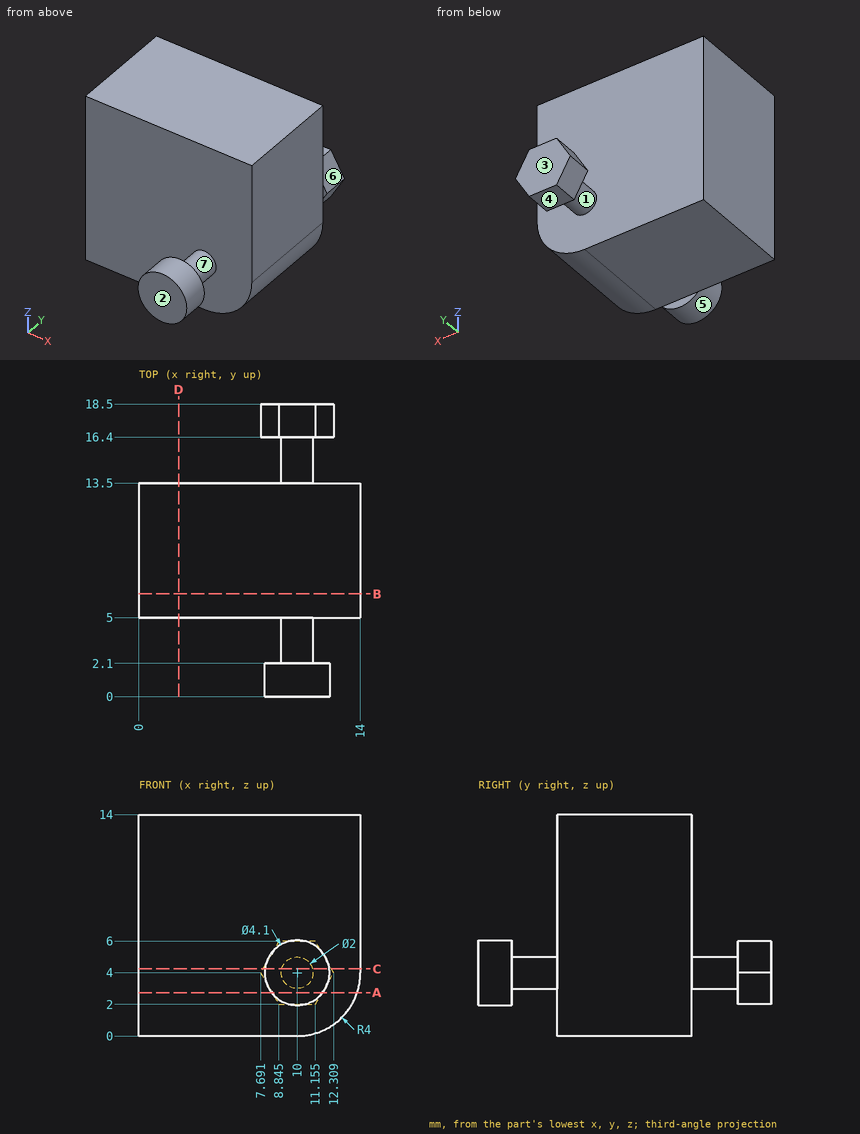
For this review, use the dimensioned drawing (mm, ordinates from the lowest corner) and the shaded views. A direction names the side the tool comes from. Round coordinates to 2 decimals unless told otherwise and drop trailing zeros. Write each loop counter-clockwise with the first axis right and the second up, starting at its lowest first coordinate (ties: lowest second). Pieces come first, ordered by that corner, then holes. Notation, with made-up numbers: (57.25, -21.5) -> (110.25, -21.5) arc R14 ccw to (110.25, -14.5) -> close; hole circle Ø11 at (-39, -23). An arc over 180 degrees is marked (long way). Answer in a Markdown table with one row per item.
Q1. Take a section at D-D, the plane x = 2.5. State the section outline as (y, z) points.
The answers:
| item | result |
|---|---|
| outline | (5, 0) -> (13.5, 0) -> (13.5, 14) -> (5, 14) -> close |
Q2. Take a section at B-B, the plane y = 6.5. State the section outline as (x, z) points, then the cut area to 3 significant figures.
The answers:
| item | result |
|---|---|
| outline | (0, 0) -> (10, 0) arc R4 ccw to (14, 4) -> (14, 14) -> (0, 14) -> close |
| area | 193 mm² |
Q3. Take a section at A-A, the plane z = 2.75. State the section outline as (x, y) points (1 decimal), then the cut area to 3 significant figures.
The answers:
| item | result |
|---|---|
| outline | (0, 5) -> (13.8, 5) -> (13.8, 13.5) -> (0, 13.5) -> close; (8.4, 0) -> (11.6, 0) -> (11.6, 2.1) -> (8.4, 2.1) -> close; (8.4, 16.4) -> (11.6, 16.4) -> (11.6, 18.5) -> (8.4, 18.5) -> close |
| area | 131 mm² |
Q4. Draft analysis for pull direction Y (two halves, no side actions). For the marked faces 1, 2 and 3, state which applies: +Y half, -Y half, draft (parallel to the pull), parting line (faces both ways), or undercut.
The answers:
| item | result |
|---|---|
| face 1 | undercut |
| face 2 | -Y half |
| face 3 | +Y half |
Q5. Clearance check with flat-ended pins moving along their axes: pin 1 Ø1.5 at (y, z) = (11.5, 2.5) entering from -X; pin 2 Ø3 at (x, y) = (9, 2) entering from -Z; pin 3 Ø1.1 at (x, y) = (10.5, 17) entering from +Z; pin 4 Ø4 at (x, z) = (4.5, 7.5) entering from +Y. State where each tip first meets the part, or that it passes through.
The answers:
| item | result |
|---|---|
| pin 1 | x = 0 |
| pin 2 | z = 1.95 |
| pin 3 | z = 6 |
| pin 4 | y = 13.5 |
Q6. To check wall thickness, follow L1, parallel to Y at x = 12.25, z = 4.5; L2, parallel to X at y = 13.25, z = 3.5; L3, parallel to Z at x = 10.25, y = 11.75. State the ranges of each line that lie inside material, in increasing order. Write a range as [from, to].
The answers:
| item | result |
|---|---|
| L1 | [5, 13.5] |
| L2 | [0, 13.97] |
| L3 | [0.01, 14] |
Q7. Take a section at C-C, the plane z = 4.25. State the section outline as (x, y) points (1 decimal).
The answers:
| item | result |
|---|---|
| outline | (0, 5) -> (9, 5) -> (9, 2.1) -> (8, 2.1) -> (8, 0) -> (12, 0) -> (12, 2.1) -> (11, 2.1) -> (11, 5) -> (14, 5) -> (14, 13.5) -> (11, 13.5) -> (11, 16.4) -> (12.2, 16.4) -> (12.2, 18.5) -> (7.8, 18.5) -> (7.8, 16.4) -> (9, 16.4) -> (9, 13.5) -> (0, 13.5) -> close |
Q8. For the marked faces 4, 5, 6 and 7, list the 3-axis set-ups (+Z, -Z, +X, -X, +Y, -Y) from which the entire face can be reached by the end or side of a thin tool; tool diameter is ignored.
The answers:
| item | result |
|---|---|
| face 4 | -Z, +X, -X, +Y |
| face 5 | -Y |
| face 6 | +Z, +X, +Y |
| face 7 | none |
